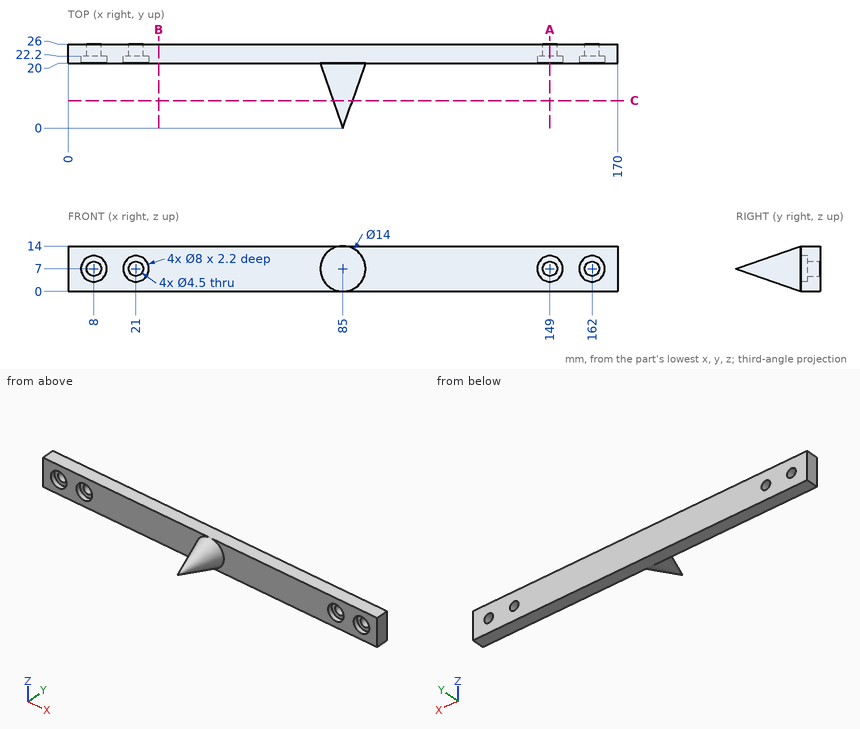
Input: dimensioned drawing with shaded views. Units: mm. Origin: part minimum x, y, z. Give positions to 0.01 mm unless a question says otherwise; leave off trailing zeros. Order: outer loops, then holes, each group sorted by start corner. A loop starts at its lowest first (then second) coordinate and runs counter-clockwise, first axis right, second up. Notation, with made-up numbers: (-5.5, 12) -> (26.5, 12) arc R27 cw to (26.5, 28) -> close; hole circle Ø8 at (-35, 76.5). An arc over 180 degrees is marked (long way). Use a Markdown table: item, result.
1) Ray query, line 1 along X through (y, z) = (21.1, 7); line 2 along Z through (x, y) = (162, 23.45); line 3 along Y through (x, z) = (33, 12.75). Return the intervals inside material, ascending. Write a range as [from, to].
Answer list:
| item | result |
|---|---|
| line 1 | [0, 4], [12, 17], [25, 145], [153, 158], [166, 170] |
| line 2 | [0, 4.75], [9.25, 14] |
| line 3 | [20, 26] |
2) Section query A-A, the plane x = 149. Return the cut outline in (y, z), then the cut area to 3 significant figures.
Answer list:
| item | result |
|---|---|
| outline | (20, 0) -> (26, 0) -> (26, 4.75) -> (22.2, 4.75) -> (22.2, 3) -> (20, 3) -> close; (20, 11) -> (22.2, 11) -> (22.2, 9.25) -> (26, 9.25) -> (26, 14) -> (20, 14) -> close |
| area | 49.3 mm² |
3) Section query B-B, the plane x = 28. Return the cut outline in (y, z).
Answer list:
| item | result |
|---|---|
| outline | (20, 0) -> (26, 0) -> (26, 14) -> (20, 14) -> close |
4) Section query C-C, the plane y = 8.5. Return the cut outline in (x, z) (3 decimals).
Answer list:
| item | result |
|---|---|
| outline | circle Ø5.95 at (85, 7) |
5) Contact query for flat-ended pins moving along their axis: P1, Ø2.5, axis at x = 8, z = 7, coming from the +Y side; P2, Ø2, axis at y = 16, z = 7.5, coming from the -X side; P3, Ø7, axis at x = 162, z = 7, coming from the -Y side; P4, Ø1, axis at y = 11.5, z = 6, coming from the -X side. Output: stop coordinate, or through.
Answer list:
| item | result |
|---|---|
| P1 | through |
| P2 | x = 79.06 |
| P3 | y = 22.2 |
| P4 | x = 80.89 |
